Part model, mm, in its own coordinate system. A direction names the side the tool comes from. Coordinates: 2 decimals unless noted, no trailing zeros. Loops run counter-clockwise (first coordinate to the right, second up) from the corner with the lowest first, then second, coordinate; pieces in that order, holes last. Notation, with made-up numbers: (-7.5, 87.25) -> (10.5, 87.25) arc R10 ccw to (10.5, 101.25) -> close; hole circle Ø9 at (-14.75, -11). An arc over 180 degrees is marked (long way). Use one line per item in the form item = value. Start each with the question number.
(1) Band-saw the part on D-D on y = -2.25. Give the cut face in (x, z).
(2) Drill centre lines: L1, parallel to Z at x = 117, y = -5.5; L2, parallel to X at y = -20, z = 12; L3, parallel to X at y = -4, z = 3. Where is each one in solid material? Low to high. Write a range as [from, to].
(3) Band-saw the part on C-C on z = 3. Give the cut face in (x, y), then the cut area to 3 significant figures.
(4) 3-axis set-ups, long thin cutter, end or side, ignore diameter. For faces 1 (the cylindrical face through (82.8, -23.95, -5.55)), 2 (the flat face through (83, -13, 5.626)), 3 (the cylindrical face through (81.8, -23.95, 4.1)), 4 (the flat face through (82, -13, -7.074)), 5 (the cylindrical face through (82.8, -1.45, -5.55)): which of +Z, -Z, +X, -X, +Y, -Y reach the whole face in a straight line?
(5) Band-saw the part on A-A on x = 60. Give the cut face in (y, z).
(6) Band-saw the part on B-B on z = 10.5. Give the cut face in (x, y), then the cut area to 3 significant figures.
(7) Mould opens along Z. For faces 6 (the cylindrical face through (20.15, -12.52, -13.8)), 7 (the cylindrical face through (81.8, -1.45, 4.1)), 8 (the flat face through (54, 0, -1)) say: +Z half, -Z half, draft (parallel to the pull), parting line (faces both ways), or undercut.
(8) Pin check, flat tips, straight feed: P1, Ø5, axis at x = 43.5, y = -4, coming from the -Z side; P2, Ø4.5, axis at x = 93.5, y = -12, coming from the -Z side; P3, Ø10, axis at x = 82, z = -8.5, coming from the -Y side; P4, Ø2, axis at x = 34.5, z = 12, coming from the -Y side. Stop position of each tip, or through.
```python
from build123d import *

# Parameters (mm, degrees)
F1_DEPTH    = 25.4
F2_F1_R     = 5.08
F2_F2_R     = 5.08
F2_F3_R     = 5.08
F2_F4_R     = 5.08
F5_T1_DEPTH = 57.4399599705
F5_T3_DEPTH = 60.5847169717


# Not quite as in the source:
# - a fillet or chamfer that OpenCascade refuses, or shapes differently, is made with other operations: its cross-section is extruded or revolved along the edge and cut away or added
# - a feature of the source that left no trace in its solid (it failed there, or was rolled back) is left out


with BuildPart() as f1:
    # F0 (on Front) → F1 (new body)
    with BuildSketch(Plane.XZ):
        with BuildLine():
            ThreePointArc((19.913375901, 8.2747844221), (44.1487619553, -0.5270852778), (20.1739600729, -10.0158007924))
            Line((20.1739600729, -10.0158007924), (17.0700166839, -12.2068939621))
            ThreePointArc((17.0700166839, -12.2068939621), (33.3560783856, -18.0313258742), (46.7383854464, -7.0735126536))
            Line((46.7383854464, -7.0735126536), (46.7383854464, 5.6264873464))
            ThreePointArc((46.7383854464, 5.6264873464), (33.4251988827, 16.5721987148), (17.1621920022, 10.8656988202))
            Line((17.1621920022, 10.8656988202), (19.913375901, 8.2747844221))
        make_face()
        with BuildLine():
            Line((46.7383854464, 5.6264873464), (46.7383854464, -7.0735126536))
            ThreePointArc((46.7383854464, -7.0735126536), (47.9263685939, -0.7235126536), (46.7383854464, 5.6264873464))
        make_face()
        with BuildLine():
            ThreePointArc((46.7383854464, 5.6264873464), (47.9263685939, -0.7235126536), (46.7383854464, -7.0735126536))
            Line((46.7383854464, -7.0735126536), (122.9383854464, -7.0735126536))
            Line((122.9383854464, -7.0735126536), (122.9383854464, 5.6264873464))
            Line((122.9383854464, 5.6264873464), (46.7383854464, 5.6264873464))
        make_face()
    extrude(amount=F1_DEPTH)

    # F2: fillet of radius 5.08 on 4 edges, made by hand

    # F2_f1
    f2_f1_edges = [f1.edges().sort_by_distance(p)[0] for p in [
        (122.9383854464, -12.7, -7.0735126536),
    ]]
    fillet(f2_f1_edges, radius=F2_F1_R)

    # F2_f2
    f2_f2_edges = [f1.edges().sort_by_distance(p)[0] for p in [
        (122.9383854464, -12.7, 5.6264873464),
    ]]
    fillet(f2_f2_edges, radius=F2_F2_R)

    # F2_f3
    f2_f3_edges = [f1.edges().sort_by_distance(p)[0] for p in [
        (122.9383854464, 0, -0.7235126536),
    ]]
    fillet(f2_f3_edges, radius=F2_F3_R)

    # F2_f4
    f2_f4_edges = [f1.edges().sort_by_distance(p)[0] for p in [
        (122.9383854464, -25.4, -0.7235126536),
    ]]
    fillet(f2_f4_edges, radius=F2_F4_R)

    # F5: fillet of radius 5.08 on 2 edges, made by hand

    # F5_s2 → F5_t1 (cut)
    with BuildSketch(Plane.XZ.offset(-16.0199799852)):
        with BuildLine():
            ThreePointArc((19.913375901, 8.2747844221), (19.7615867452, 12.0028035456), (22.1975397768, 14.8289846016))
            ThreePointArc((22.1975397768, 14.8289846016), (19.4976030488, 13.0789063368), (17.1621920022, 10.8656988202))
            Line((17.1621920022, 10.8656988202), (19.913375901, 8.2747844221))
        make_face()
    extrude(amount=F5_T1_DEPTH, mode=Mode.SUBTRACT)

    # F5_s4 → F5_t3 (cut)
    with BuildSketch(Plane.XZ.offset(-17.5923584858)):
        with BuildLine():
            ThreePointArc((22.6439130786, -16.5022695354), (20.1284364115, -13.7466310122), (20.1739600729, -10.0158007924))
            Line((20.1739600729, -10.0158007924), (17.0700166839, -12.2068939621))
            ThreePointArc((17.0700166839, -12.2068939621), (19.6396592089, -14.6365685699), (22.6439130786, -16.5022695354))
        make_face()
    extrude(amount=F5_T3_DEPTH, mode=Mode.SUBTRACT)


solid = f1.part
```
A:
q1.outline = (19.91, 8.27) arc R13.79 cw (long way) to (20.17, -10.02) arc R5.08 ccw to (22.64, -16.5) arc R17.56 ccw to (47.05, -6.21) -> (117.86, -6.21) arc R4.22 ccw to (122.08, -1.99) -> (122.08, 0.55) arc R4.22 ccw to (117.86, 4.77) -> (47.05, 4.77) arc R17.56 ccw to (22.2, 14.83) arc R5.08 ccw to start
q2.L1 = [-7.07, 5.63]
q2.L2 = [19.76, 25.05], [35.68, 42.47]
q2.L3 = [43.64, 122.17]
q3.outline = (43.64, -25.4) -> (47.53, -25.4) -> (47.53, -24.77) -> (117.86, -24.77) arc R4.45 ccw to (122.31, -20.32) -> (122.31, -5.08) arc R4.45 ccw to (117.86, -0.63) -> (47.53, -0.63) -> (47.53, 0) -> (43.64, 0) -> close
q3.area = 1,900 mm²
q4.face_1 = -Z, +X, -Y
q4.face_2 = +Z, +X, +Y, -Y
q4.face_3 = +Z, +X, -Y
q4.face_4 = -Z, +X, +Y, -Y
q4.face_5 = -Z, +X, +Y
q5.outline = (-25.4, -1.99) arc R5.08 ccw to (-20.32, -7.07) -> (-5.08, -7.07) arc R5.08 ccw to (0, -1.99) -> (0, 0.55) arc R5.08 ccw to (-5.08, 5.63) -> (-20.32, 5.63) arc R5.08 ccw to (-25.4, 0.55) -> close
q6.outline = (19.48, -25.4) -> (22.35, -25.4) -> (22.35, 0) -> (19.48, 0) -> close; (38.37, -25.4) -> (43.87, -25.4) -> (43.87, 0) -> (38.37, 0) -> close
q6.area = 213 mm²
q7.face_6 = undercut
q7.face_7 = +Z half
q7.face_8 = draft
q8.P1 = -14.7
q8.P2 = -7.07
q8.P3 = -25.17
q8.P4 = -25.4
